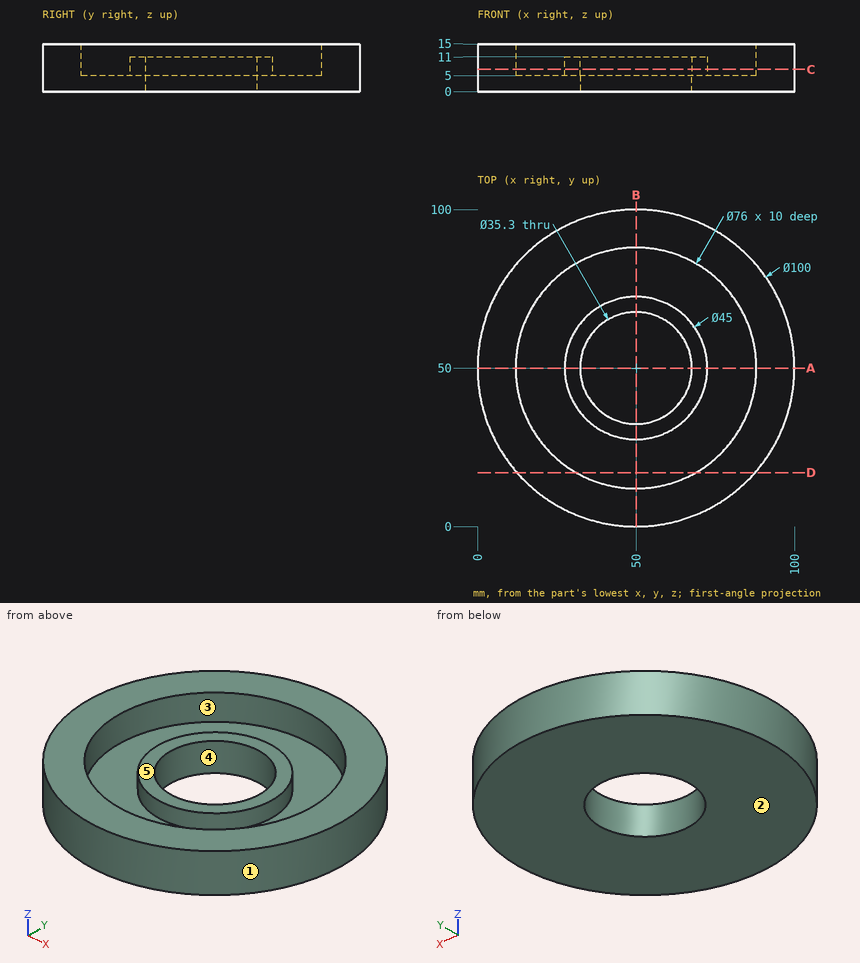
Answer from the drawing. Dimensions are ordinates in mm from the lowest x, y and z of the part. A direction names the side the tool comes from. Round coordinates to 2 decimals unless told otherwise and drop trailing zeros. Write each loop counter-clockwise with the first axis right and the second up, starting at its lowest first coordinate (ties: lowest second). Pieces come first, ordered by that corner, then holes. Notation, with made-up numbers: (9.5, 67.25) - (17.5, 67.25) arc R34 ccw to (17.5, 102.25) - close; hole circle Ø8 at (-17.75, -40). An arc over 180 degrees is marked (long way). Use a Markdown table: item, result.
(1) Which of the six approach directions +Z, -Z, +X, -X, +Y, -Y give full straight-line access (tool end or side, diameter ignored) to the marked faces 4 and 5?
Reported:
| item | result |
|---|---|
| face 4 | +Z, -Z |
| face 5 | +Z |
(2) Each of these flat-tipped pins is pushed along its axis until it touches: pin 1 Ø8 at (x, z) = (51.5, 3.5) entering from +Y; pin 2 Ø6 at (y, z) = (62, 8) entering from -X; pin 3 Ø12 at (x, y) = (65, 59.5) entering from +Z; pin 4 Ø8 at (x, y) = (58.5, 58.5) entering from +Z. Where does it stop, or does it pass through?
Reported:
| item | result |
|---|---|
| pin 1 | y = 100 |
| pin 2 | x = 0.82 |
| pin 3 | z = 11 |
| pin 4 | through |
(3) The part is cut by section C-C (z = 7). Write down the section's boundary in (x, y).
Reported:
| item | result |
|---|---|
| outline | circle Ø100 at (50, 50); circle Ø45 at (50, 50); hole circle Ø76 at (50, 50); hole circle Ø35.3 at (50, 50) |
(4) The part is cut by section A-A (y = 50). Write down the section's boundary in (x, z).
Reported:
| item | result |
|---|---|
| outline | (0, 0) - (32.35, 0) - (32.35, 11) - (27.5, 11) - (27.5, 5) - (12, 5) - (12, 15) - (0, 15) - close; (67.65, 0) - (100, 0) - (100, 15) - (88, 15) - (88, 5) - (72.5, 5) - (72.5, 11) - (67.65, 11) - close |
(5) Straight lines are drawn through the part: line 1 along Y through (x, z) = (50, 11.75); line 2 along X through (y, z) = (35, 6); line 3 along X through (y, z) = (37.5, 8.25). For each, find the intervals that lie inside material, in ascending order. Write a range as [from, to].
Reported:
| item | result |
|---|---|
| line 1 | [0, 12], [88, 100] |
| line 2 | [2.3, 15.09], [33.23, 40.7], [59.3, 66.77], [84.91, 97.7] |
| line 3 | [1.59, 14.11], [31.29, 37.54], [62.46, 68.71], [85.89, 98.41] |
(6) The part is cut by section D-D (y = 17). Write down the section's boundary in (x, z), then the cut area to 3 significant figures.
Reported:
| item | result |
|---|---|
| outline | (12.44, 0) - (87.56, 0) - (87.56, 15) - (68.84, 15) - (68.84, 5) - (31.16, 5) - (31.16, 15) - (12.44, 15) - close |
| area | 750 mm2 |
(7) The mould has two halves that part along Y. Classify the marked faces 1, 2 and 3: released by +Y, released by -Y, zero draft, split by the parting line, or undercut.
Reported:
| item | result |
|---|---|
| face 1 | split by the parting line |
| face 2 | zero draft |
| face 3 | undercut |
